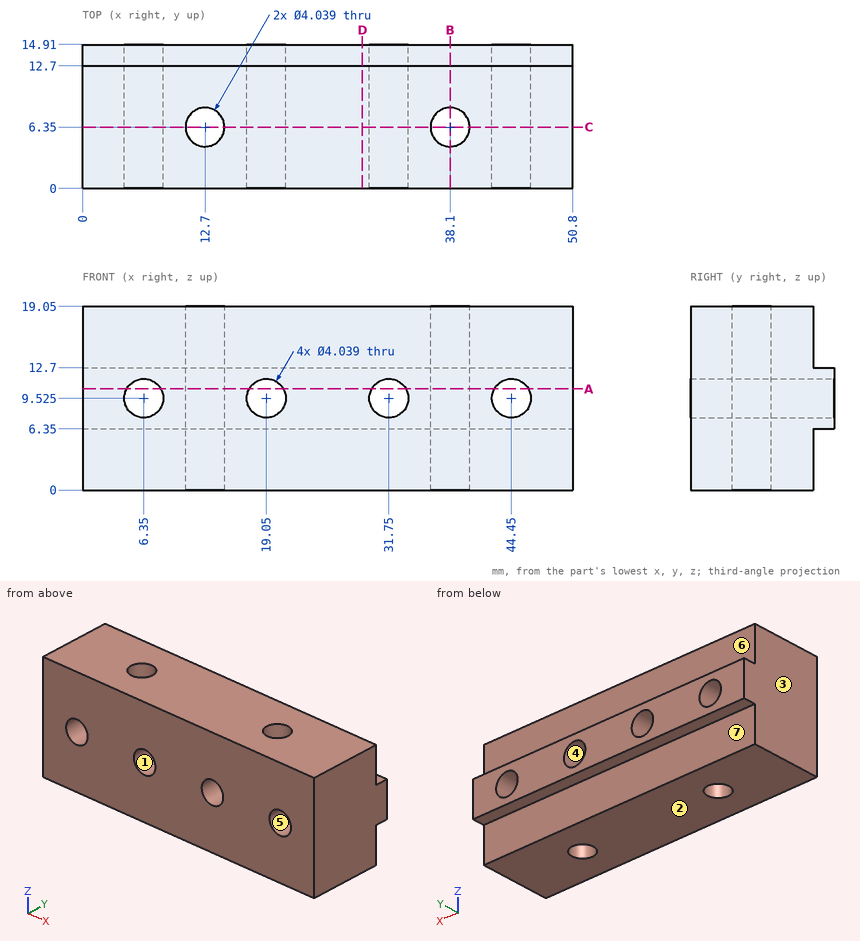
Here's the drawing with two shaded views (mm, measured from the low corner). I have some questions. A direction names the side the tool comes from. Coordinates: 2 decimals unless noted, no trailing zeros. Loops run counter-clockwise (first coordinate to the right, second up) from the corner with the lowest first, then second, coordinate; pieces in that order, holes last.
Item 1: Suppose I cut it at A-A (z = 10.5). Please give me the cut outline in (x, y), then the cut area to 3 significant figures.
Answers below:
outline: (0, 0) - (4.58, 0) - (4.58, 14.91) - (0, 14.91) - close; (8.12, 0) - (17.28, 0) - (17.28, 14.91) - (8.12, 14.91) - close; (20.82, 0) - (29.98, 0) - (29.98, 14.91) - (20.82, 14.91) - close; (33.52, 0) - (42.68, 0) - (42.68, 14.91) - (33.52, 14.91) - close; (46.22, 0) - (50.8, 0) - (50.8, 14.91) - (46.22, 14.91) - close; hole circle Ø4.04 at (12.7, 6.35); hole circle Ø4.04 at (38.1, 6.35)
area: 521 mm2
Item 2: I'm going to push flat-ended pins straight in: pin 1 (2.5 mm diameter, centred on x = 12.7, y = 6.35, fed in from -Z); pin 2 (5 mm diameter, centred on x = 27.5, z = 17.5, fed in from +Y). Where does each tip first touch, or does it pass through?
Answers below:
pin 1: passes through
pin 2: stops at y = 12.7
Item 3: Please list where these lines run through material, in increasing order: L1, parallel to X at y = 6.5, z = 1.25; L2, parallel to X at y = 4, z = 8 (1 decimal); L3, parallel to Y at x = 38.1, z = 9.75.
Answers below:
L1: x = 0 to 10.69, 14.71 to 36.09, 40.11 to 50.8
L2: x = 0 to 5, 7.7 to 17.7, 20.4 to 30.4, 33.1 to 43.1, 45.8 to 50.8
L3: y = 0 to 4.33, 8.37 to 14.91
Item 4: Suppose I cut it at D-D (x = 29). Please give me the cut outline in (y, z), then the cut area to 3 significant figures.
Answers below:
outline: (0, 0) - (12.7, 0) - (12.7, 6.35) - (14.91, 6.35) - (14.91, 12.7) - (12.7, 12.7) - (12.7, 19.05) - (0, 19.05) - close
area: 256 mm2
Item 5: If we mould it in two halves opening along X, with no side actions, what happens to the marked faces 1, 2, 3 and 4? For each: released by +X, released by -X, zero draft, split by the parting line, or undercut.
Answers below:
face 1: undercut
face 2: zero draft
face 3: released by -X
face 4: undercut
Item 6: Suppose I cut it at C-C (y = 6.35). State how many separate pieces and enclosed holes the cut face has.
Answers below:
separate pieces: 3
enclosed holes: 4
Item 7: Which directions (+Z, -Z, +X, -X, +Y, -Y) give clear straight access to the entire face, cutting with the end or side of a thin tool? Please do the marked faces 5, 6 and 7.
Answers below:
face 5: +Y, -Y
face 6: +Z, +X, -X, +Y
face 7: -Z, +X, -X, +Y
Item 8: Suppose I cut it at B-B (x = 38.1). Please give me the cut outline in (y, z).
Answers below:
outline: (0, 0) - (4.33, 0) - (4.33, 19.05) - (0, 19.05) - close; (8.37, 0) - (12.7, 0) - (12.7, 6.35) - (14.91, 6.35) - (14.91, 12.7) - (12.7, 12.7) - (12.7, 19.05) - (8.37, 19.05) - close
